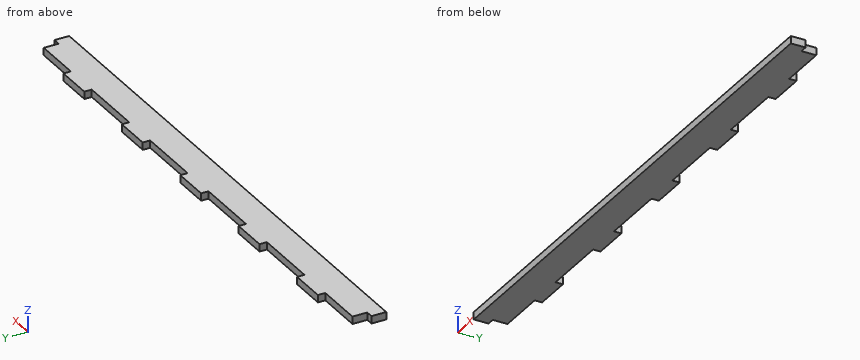
from build123d import *

# Parameters (mm, degrees)
BOSS_EXTRUDE1_DEPTH = 2.5


with BuildPart() as part:
    # Sketch1 → Boss-Extrude1 (new, symmetric)
    with BuildSketch(Plane.XY):
        Polygon((410, -35), (410, -25), (377.5, -25), (377.5, -20), (352.5, -20), (352.5, -25), (307.5, -25), (307.5, -20), (282.5, -20), (282.5, -25), (237.5, -25), (237.5, -20), (212.5, -20), (212.5, -25), (167.5, -25), (167.5, -20), (142.5, -20), (142.5, -25), (97.5, -25), (97.5, -20), (72.5, -20), (72.5, -25), (40, -25), (40, -35), (35, -35), (35, -45), (40, -45), (410, -45), (415, -45), (415, -35), align=None)
    extrude(amount=BOSS_EXTRUDE1_DEPTH, both=True)


solid = part.part
Read the model definition and answer for the solid it produces. Units are mm, in the model's axes. Give positions to 0.01 mm unless a question says otherwise; leave off trailing zeros. Loops run counter-clockwise (first coordinate to the right, second up) from the corner with the lowest first, then second, coordinate; pieces in that order, holes last. Notation, with made-up numbers: (36.5, -8.75) -> (81.5, -8.75) arc R21 ccw to (81.5, 5.25) -> close; hole circle Ø6 at (12, 54.5). An arc over 180 degrees is marked (long way). Answer as CSV lines item,"result".
Item 1: Each of these flat-tipped pins is pushed along its axis until it touches: pin 1 (2.5 mm diameter, centred on y = -23, z = -0.5, fed in from -X); pin 2 (2 mm diameter, centred on y = -26, z = -1, fed in from -X); pin 3 (2.5 mm diameter, centred on y = -32.5, z = 1, fed in from +X). Where does it stop, or does it pass through?
Returned:
pin 1,"stops at x = 72.5"
pin 2,"stops at x = 40"
pin 3,"stops at x = 410"
Item 2: Find section A-A on z = -0.25. Give the vertices of the cut face in (x, y), plus the area to 4 significant figures.
Returned:
outline,"(35, -45) -> (415, -45) -> (415, -35) -> (410, -35) -> (410, -25) -> (377.5, -25) -> (377.5, -20) -> (352.5, -20) -> (352.5, -25) -> (307.5, -25) -> (307.5, -20) -> (282.5, -20) -> (282.5, -25) -> (237.5, -25) -> (237.5, -20) -> (212.5, -20) -> (212.5, -25) -> (167.5, -25) -> (167.5, -20) -> (142.5, -20) -> (142.5, -25) -> (97.5, -25) -> (97.5, -20) -> (72.5, -20) -> (72.5, -25) -> (40, -25) -> (40, -35) -> (35, -35) -> close"
area,"8,125 mm²"
Item 3: Find section C-C on y = -31. Give the vertices of the cut face in (x, z), plus the area to 3 significant figures.
Returned:
outline,"(40, -2.5) -> (410, -2.5) -> (410, 2.5) -> (40, 2.5) -> close"
area,"1,850 mm²"
Item 4: Consider line 1 (Y direction, x = 120, z = 1.9); line 2 (X direction, y = -31, z = -1.25). Determine where each line is inside the solid, lowest interval first. Write a range as [from, to].
Returned:
line 1,"y = [-45, -25]"
line 2,"x = [40, 410]"
Item 5: Find section B-B on x = 324.5. Give the vertices of the cut face in (y, z).
Returned:
outline,"(-45, -2.5) -> (-25, -2.5) -> (-25, 2.5) -> (-45, 2.5) -> close"
